Here's how the part is built. I have some questions about the finished solid (model axes, mm). Round coordinates to 2 decimals unless told otherwise and drop trailing zeros. Order: outer loops, then holes, each group sorted by start corner. A loop starts at its lowest first (then second) coordinate and runs counter-clockwise, first axis right, second up.
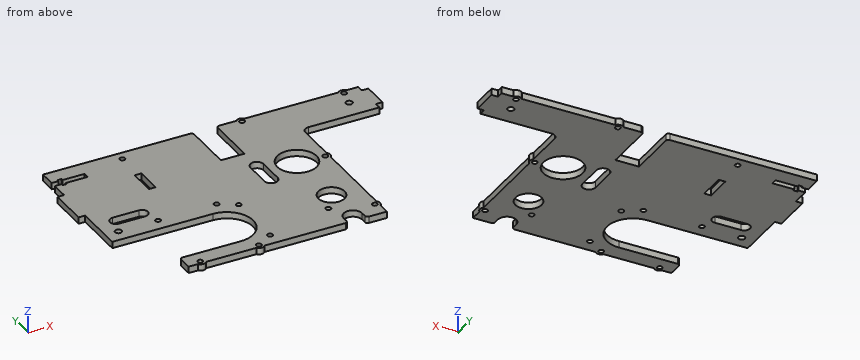
```python
from build123d import *

# Parameters (mm, degrees)
SKETCH1_W                = 240
SKETCH1_H                = 151
BOSS_EXTRUDE1_DEPTH      = 5
SKETCH5_R                = 2
CUT_EXTRUDE1_DEPTH       = 5
SKETCH6_R                = 4
SKETCH6_R_2              = 2
BOSS_EXTRUDE2_DEPTH      = 5
CUT_EXTRUDE2_DEPTH       = 5
SKETCH8_W                = 30
SKETCH8_H                = 12.5
CUT_EXTRUDE3_DEPTH       = 5
SKETCH9_W                = 59
SKETCH9_H                = 121
CUT_EXTRUDE4_DEPTH       = 5
SKETCH12_W               = 18
SKETCH12_H               = 40
CUT_EXTRUDE7_DEPTH       = 10
SKETCH13_R               = 2
CUT_EXTRUDE8_DEPTH       = 10
SKETCH15_R               = 2
CUT_EXTRUDE9_DEPTH       = 5
SKETCH16_W               = 5.2
SKETCH16_H               = 20.2
CUT_EXTRUDE10_DEPTH      = 5
SKETCH17_R               = 4
SKETCH17_R_2             = 2
BOSS_EXTRUDE3_DEPTH      = 5
CUT_EXTRUDE11_DEPTH      = 10
SKETCH19_R               = 15
CUT_EXTRUDE12_DEPTH      = 10
CUT_EXTRUDE13_DEPTH      = 1
CUT_EXTRUDE13_DEPTH_BACK = 10
SKETCH23_R               = 2
CUT_EXTRUDE16_DEPTH      = 5
SKETCH24_R               = 4
SKETCH24_R_2             = 2
BOSS_EXTRUDE4_DEPTH      = 5
SKETCH27_R               = 2.5
CUT_EXTRUDE18_DEPTH      = 10
CUT_EXTRUDE19_DEPTH      = 10
SKETCH31_R               = 2.5
CUT_EXTRUDE20_DEPTH      = 10
SKETCH32_W               = 5
SKETCH32_H               = 30
SKETCH32_H_2             = 20
BOSS_EXTRUDE6_DEPTH      = 5
FILLET1_R                = 5
FILLET2_R                = 2
CUT_EXTRUDE22_DEPTH      = 5
SKETCH35_R               = 10
CUT_EXTRUDE23_DEPTH      = 5
SKETCH36_R               = 2
CUT_EXTRUDE24_DEPTH      = 5


with BuildPart() as part:
    # Sketch1 → Boss-Extrude1 (new body)
    with BuildSketch(Plane.XY):
        Rectangle(SKETCH1_W, SKETCH1_H)
    extrude(amount=BOSS_EXTRUDE1_DEPTH)

    # Sketch5 → Cut-Extrude1 (cut)
    with BuildSketch(Plane(origin=(0, 0, 0), x_dir=(-1, 0, 0), z_dir=(0, 0, -1))):
        with Locations((35.2, -73)):
            Circle(SKETCH5_R)
        with Locations((79.8, -73)):
            Circle(SKETCH5_R)
        with Locations((22.5, -65.3)):
            Circle(SKETCH5_R)
        with Locations((22.5, -20.7)):
            Circle(SKETCH5_R)
        with Locations((79.8, -13)):
            Circle(SKETCH5_R)
        with Locations((35.2, -13)):
            Circle(SKETCH5_R)
    extrude(amount=-CUT_EXTRUDE1_DEPTH, mode=Mode.SUBTRACT)

    # Sketch6 → Boss-Extrude2 (add)
    with BuildSketch(Plane(origin=(0, 0, 0), x_dir=(-1, 0, 0), z_dir=(0, 0, -1))):
        with Locations((35.2, -73)):
            Circle(SKETCH6_R)
        with Locations((35.2, -73)):
            Circle(SKETCH6_R_2, mode=Mode.SUBTRACT)
        with Locations((79.8, -73)):
            Circle(SKETCH6_R)
        with Locations((79.8, -73)):
            Circle(SKETCH6_R_2, mode=Mode.SUBTRACT)
    extrude(amount=-BOSS_EXTRUDE2_DEPTH)

    # Sketch7 → Cut-Extrude2 (cut)
    with BuildSketch(Plane(origin=(0, 0, 0), x_dir=(-1, 0, 0), z_dir=(0, 0, -1))):
        with BuildLine():
            Line((120, -63), (43.5, -63))
            ThreePointArc((43.5, -63), (23.5, -43), (43.5, -23))
            Line((43.5, -23), (120, -23))
            Line((120, -23), (120, -63))
        make_face()
    extrude(amount=-CUT_EXTRUDE2_DEPTH, mode=Mode.SUBTRACT)

    # Sketch8 → Cut-Extrude3 (cut)
    with BuildSketch(Plane(origin=(0, 0, 0), x_dir=(-1, 0, 0), z_dir=(0, 0, -1))):
        with Locations((105, -69.25)):
            Rectangle(SKETCH8_W, SKETCH8_H)
    extrude(amount=-CUT_EXTRUDE3_DEPTH, mode=Mode.SUBTRACT)

    # Sketch9 → Cut-Extrude4 (cut)
    with BuildSketch(Plane(origin=(0, 0, 0), x_dir=(-1, 0, 0), z_dir=(0, 0, -1))):
        with Locations((-90.5, -15)):
            Rectangle(SKETCH9_W, SKETCH9_H)
    extrude(amount=-CUT_EXTRUDE4_DEPTH, mode=Mode.SUBTRACT)

    # Sketch12 → Cut-Extrude7 (cut)
    with BuildSketch(Plane(origin=(0, 0, 0), x_dir=(-1, 0, 0), z_dir=(0, 0, -1))):
        with Locations((-3, 55.5)):
            Rectangle(SKETCH12_W, SKETCH12_H)
    extrude(amount=-CUT_EXTRUDE7_DEPTH, mode=Mode.SUBTRACT)

    # Sketch13 → Cut-Extrude8 (cut)
    with BuildSketch(Plane(origin=(0, 0, 0), x_dir=(-1, 0, 0), z_dir=(0, 0, -1))):
        with Locations((-58.295562695, 7.3)):
            Circle(SKETCH13_R)
        with Locations((-58.295562695, -63.3)):
            Circle(SKETCH13_R)
    extrude(amount=-CUT_EXTRUDE8_DEPTH, mode=Mode.SUBTRACT)

    # Sketch15 → Cut-Extrude9 (cut)
    with BuildSketch(Plane.XY.offset(5)):
        with Locations((-63.5, 68.3)):
            Circle(SKETCH15_R)
    extrude(amount=-CUT_EXTRUDE9_DEPTH, mode=Mode.SUBTRACT)

    # Sketch16 → Cut-Extrude10 (cut)
    with BuildSketch(Plane(origin=(0, 0, 0), x_dir=(-1, 0, 0), z_dir=(0, 0, -1))):
        with Locations((63.6, 35.6)):
            Rectangle(SKETCH16_W, SKETCH16_H)
    extrude(amount=-CUT_EXTRUDE10_DEPTH, mode=Mode.SUBTRACT)

    # Sketch17 → Boss-Extrude3 (add)
    with BuildSketch(Plane(origin=(0, 0, 0), x_dir=(-1, 0, 0), z_dir=(0, 0, -1))):
        with Locations((-58.295562695, 7.3)):
            Circle(SKETCH17_R)
        with Locations((-58.295562695, 7.3)):
            Circle(SKETCH17_R_2, mode=Mode.SUBTRACT)
        with Locations((-58.295562695, -63.3)):
            Circle(SKETCH17_R)
        with Locations((-58.295562695, -63.3)):
            Circle(SKETCH17_R_2, mode=Mode.SUBTRACT)
    extrude(amount=-BOSS_EXTRUDE3_DEPTH)

    # Sketch18 → Cut-Extrude11 (cut)
    with BuildSketch(Plane(origin=(0, 0, 0), x_dir=(-1, 0, 0), z_dir=(0, 0, -1))):
        with BuildLine():
            Line((-7.007007892, 17.8501367), (-7.007007892, -2.1498633))
            ThreePointArc((-7.007007892, -2.1498633), (-12.007007892, -7.1498633), (-17.007007892, -2.1498633))
            Line((-17.007007892, -2.1498633), (-17.007007892, 17.8501367))
            ThreePointArc((-17.007007892, 17.8501367), (-12.007007892, 22.8501367), (-7.007007892, 17.8501367))
        make_face()
    extrude(amount=-CUT_EXTRUDE11_DEPTH, mode=Mode.SUBTRACT)

    # Sketch19 → Cut-Extrude12 (cut)
    with BuildSketch(Plane(origin=(0, 0, 0), x_dir=(-1, 0, 0), z_dir=(0, 0, -1))):
        with Locations((-38.295562695, 10.103446171)):
            Circle(SKETCH19_R)
    extrude(amount=-CUT_EXTRUDE12_DEPTH, mode=Mode.SUBTRACT)

    # Sketch20 → Cut-Extrude13 (cut, two sides)
    with BuildSketch(Plane(origin=(0, 0, 0), x_dir=(-1, 0, 0), z_dir=(0, 0, -1))) as cut_extrude13_sk:
        with BuildLine():
            ThreePointArc((-31.295562695, -69.5), (-38.295562695, -62.5), (-45.295562695, -69.5))
            Line((-45.295562695, -69.5), (-45.295562695, -75.5))
            Line((-45.295562695, -75.5), (-31.295562695, -75.5))
            Line((-31.295562695, -75.5), (-31.295562695, -69.5))
        make_face()
    extrude(amount=CUT_EXTRUDE13_DEPTH, mode=Mode.SUBTRACT)
    extrude(cut_extrude13_sk.sketch, amount=-CUT_EXTRUDE13_DEPTH_BACK, mode=Mode.SUBTRACT)

    # Sketch23 → Cut-Extrude16 (cut)
    with BuildSketch(Plane(origin=(0, 0, 0), x_dir=(-1, 0, 0), z_dir=(0, 0, -1))):
        with Locations((-107.8, 73)):
            Circle(SKETCH23_R)
        with Locations((-30.2, 73)):
            Circle(SKETCH23_R)
    extrude(amount=-CUT_EXTRUDE16_DEPTH, mode=Mode.SUBTRACT)

    # Sketch24 → Boss-Extrude4 (add)
    with BuildSketch(Plane(origin=(0, 0, 0), x_dir=(-1, 0, 0), z_dir=(0, 0, -1))):
        with Locations((-107.8, 73)):
            Circle(SKETCH24_R)
        with Locations((-107.8, 73)):
            Circle(SKETCH24_R_2, mode=Mode.SUBTRACT)
        with Locations((-30.2, 73)):
            Circle(SKETCH24_R)
        with Locations((-30.2, 73)):
            Circle(SKETCH24_R_2, mode=Mode.SUBTRACT)
    extrude(amount=-BOSS_EXTRUDE4_DEPTH)

    # Sketch27 → Cut-Extrude18 (cut)
    with BuildSketch(Plane(origin=(0, 0, 0), x_dir=(-1, 0, 0), z_dir=(0, 0, -1))):
        with Locations((110, -13)):
            Circle(SKETCH27_R)
    extrude(amount=-CUT_EXTRUDE18_DEPTH, mode=Mode.SUBTRACT)

    # Sketch30 → Cut-Extrude19 (cut)
    with BuildSketch(Plane(origin=(0, 0, 0), x_dir=(-1, 0, 0), z_dir=(0, 0, -1))):
        with BuildLine():
            Line((105, -4.424095919), (85, -4.424095919))
            ThreePointArc((85, -4.424095919), (80.575904081, 0), (85, 4.424095919))
            Line((85, 4.424095919), (105, 4.424095919))
            ThreePointArc((105, 4.424095919), (109.424095919, 0), (105, -4.424095919))
        make_face()
    extrude(amount=-CUT_EXTRUDE19_DEPTH, mode=Mode.SUBTRACT)

    # Sketch31 → Cut-Extrude20 (cut)
    with BuildSketch(Plane(origin=(0, 0, 0), x_dir=(-1, 0, 0), z_dir=(0, 0, -1))):
        with Locations((-105, 60.5)):
            Circle(SKETCH31_R)
    extrude(amount=-CUT_EXTRUDE20_DEPTH, mode=Mode.SUBTRACT)

    # Sketch32 → Boss-Extrude6 (add)
    with BuildSketch(Plane(origin=(0, 0, 0), x_dir=(-1, 0, 0), z_dir=(0, 0, -1))):
        with Locations((122.5, 30.5)):
            Rectangle(SKETCH32_W, SKETCH32_H)
        with Locations((-122.5, 60.5)):
            Rectangle(SKETCH32_W, SKETCH32_H_2)
    extrude(amount=-BOSS_EXTRUDE6_DEPTH)

    # Fillet1
    fillet1_edges = [part.edges().sort_by_distance(p)[0] for p in [
        (61, 45.5, 2.5),
    ]]
    fillet(fillet1_edges, radius=FILLET1_R)

    # Fillet2
    fillet2_edges = [part.edges().sort_by_distance(p)[0] for p in [
        (12, 75.5, 2.5),
        (-6, 75.5, 2.5),
        (31.295562695, -75.5, 2.5),
        (45.295562695, -75.5, 2.5),
        (-90, -63, 2.5),
    ]]
    fillet(fillet2_edges, radius=FILLET2_R)

    # Sketch34 → Cut-Extrude22 (cut)
    with BuildSketch(Plane(origin=(0, 0, 0), x_dir=(-1, 0, 0), z_dir=(0, 0, -1))):
        Polygon((115, 58.736739195), (120, 58.736739195), (120, 63.136739195), (115, 63.136739195), (115, 64.636739195), (111.7, 64.636739195), (111.7, 63.136739195), (95, 63.136739195), (95, 58.736739195), (111.7, 58.736739195), (111.7, 57.236739195), (115, 57.236739195), align=None)
    extrude(amount=-CUT_EXTRUDE22_DEPTH, mode=Mode.SUBTRACT)

    # Sketch35 → Cut-Extrude23 (cut)
    with BuildSketch(Plane(origin=(0, 0, 0), x_dir=(-1, 0, 0), z_dir=(0, 0, -1))):
        with Locations((-38.295562695, -38.978399319)):
            Circle(SKETCH35_R)
    extrude(amount=-CUT_EXTRUDE23_DEPTH, mode=Mode.SUBTRACT)

    # Sketch36 → Cut-Extrude24 (cut)
    with BuildSketch(Plane(origin=(0, 0, 0), x_dir=(-1, 0, 0), z_dir=(0, 0, -1))):
        with Locations((-28.16035742, -53.440416767)):
            Circle(SKETCH36_R)
    extrude(amount=-CUT_EXTRUDE24_DEPTH, mode=Mode.SUBTRACT)


solid = part.part
```
1. I need wall thicknesses on probe 1 along X at (y, z) = (68.5, 3.95); probe 2 along Y at (x, z) = (-103.5, 3.1); probe 3 along X at (y, z) = (-2.5, 2.45). Which ranges of each line are inside material? Lowest first, please.
Evaluation:
probe 1: x = -120 to -65.49, -61.51 to -6, 12 to 125
probe 2: y = -23 to -4.42, 4.42 to 58.74, 63.14 to 75.5
probe 3: x = -120 to -108.65, -81.35 to 7.02, 16.99 to 30.16, 46.43 to 61
2. If we section it at A-A, the plane y = 0.5: Write out the boundary of the cut face in (x, z).
Evaluation:
outline: (-120, 0) - (-109.4, 0) - (-109.4, 5) - (-120, 5) - close; (-80.6, 0) - (7.01, 0) - (7.01, 5) - (-80.6, 5) - close; (17.01, 0) - (26.77, 0) - (26.77, 5) - (17.01, 5) - close; (49.82, 0) - (61, 0) - (61, 5) - (49.82, 5) - close
3. If we section it at D-D, the plane z = 1.5: State how many separate pieces and enclosed holes the cut face has, and give its area (3 significant figures).
Evaluation:
separate pieces: 1
enclosed holes: 19
area: 22,500 mm2
4. I'm going to push flat-ended pins straight in: P1, Ø1.5, axis at y = -1.5, z = 1.5, coming from the -X side; P2, Ø1.5, axis at x = -60.5, z = 2, coming from the +Y side; P3, Ø1, axis at x = 17, z = 4, coming from the -Y side; P4, Ø2.5, axis at x = -22.5, y = -65.3, coming from the -Z side. Where does each tip first touch, or does it pass through?
Evaluation:
P1: stops at x = -120
P2: stops at y = 75.5
P3: stops at y = -75.5
P4: passes through
5. If we section it at B-B, the plane x = 37: Write out the boundary of the cut face in (y, z), and give its area (3 significant figures).
Evaluation:
outline: (-62.62, 0) - (-48.89, 0) - (-48.89, 5) - (-62.62, 5) - close; (-29.06, 0) - (-4.84, 0) - (-4.84, 5) - (-29.06, 5) - close; (25.05, 0) - (75.5, 0) - (75.5, 5) - (25.05, 5) - close
area: 442 mm2
6. If we section it at C-C, the plane x = -12.5: Write out the boundary of the cut face in (y, z), and give its area (3 significant figures).
Evaluation:
outline: (-75.5, 0) - (75.5, 0) - (75.5, 5) - (-75.5, 5) - close
area: 755 mm2
